For this review, take the finished solid that the model builds, in its own axes (mm). Face numbers are marked on the shaded views. A direction names the side the tool comes from. Round coordinates to 2 decimals unless told otherwise and drop trailing zeros. Write each loop counter-clockwise with the first axis right and the second up, starting at its lowest first coordinate (ties: lowest second). Pieces come first, ordered by that corner, then holes. Notation, with made-up numbers: (27, -14.75) -> (63, -14.75) arc R21 ccw to (63, 24.25) -> close; hole circle Ø9 at (4, -31). An arc over 180 degrees is marked (long way). Answer in a Markdown table with one row per item.
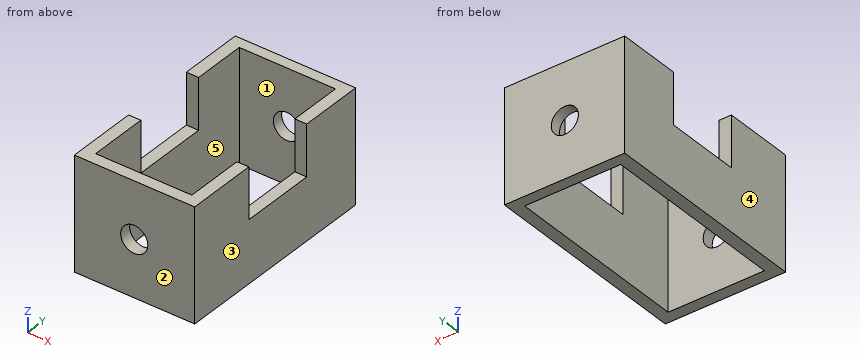
from build123d import *

# Parameters (mm, degrees)
F0_W     = 106.1013787985
F0_H     = 185.8578324318
F1_DEPTH = 99.4051918387
F2_R     = 11.9577926149
F3_DEPTH = 185.8588324318
F4_W     = 66.8169781566
F4_H     = 44.8713488877
F5_DEPTH = 106.1023787985
F6_W     = 84.8165526986
F6_H     = 165.8911928535
F7_DEPTH = 99.4061918387


with BuildPart() as f1:
    # F0 (on Top) → F1 (new body)
    with BuildSketch(Plane.XY):
        with Locations((-35.3671237826, 0)):
            Rectangle(F0_W, F0_H)
    extrude(amount=F1_DEPTH)

    # F2 (on face) → F3 (cut, through all)
    with BuildSketch(Plane.XZ.offset(92.9289162159)):
        with Locations((-35.6283932924, 49.7025959194)):
            Circle(F2_R)
    extrude(amount=-F3_DEPTH, mode=Mode.SUBTRACT)

    # F4 (on face) → F5 (cut, through all)
    with BuildSketch(Plane(origin=(-88.4178131819, 0, 0), x_dir=(0, -1, 0), z_dir=(-1, 0, 0))):
        with Locations((-3.043372184, 76.9695173949)):
            Rectangle(F4_W, F4_H)
    extrude(amount=-F5_DEPTH, mode=Mode.SUBTRACT)

    # F6 (on face) → F7 (cut, through all)
    with BuildSketch(Plane.XY.offset(99.4051918387)):
        with Locations((-35.2126248181, 0.4157535732)):
            Rectangle(F6_W, F6_H)
    extrude(amount=-F7_DEPTH, mode=Mode.SUBTRACT)


solid = f1.part
1) Mouldability with a two-part tool opening along X and no side actions: class the marked faces 1, 2 and 3 as pulls with the +X half, pulls with the -X half, needs draft (parallel to the pull), parting line crosses it, or undercut.
Solved:
| item | result |
|---|---|
| face 1 | undercut |
| face 2 | needs draft |
| face 3 | pulls with the +X half |
2) Clearance check with flat-ended pins moving along their axes: pin 1 Ø10 at (y, z) = (21, 64) entering from +X; pin 2 Ø8.5 at (x, y) = (14, 4) entering from +Z. State where each tip first meets the part, or that it passes through.
Solved:
| item | result |
|---|---|
| pin 1 | through |
| pin 2 | z = 54.53 |
3) For the marked faces 4 and 5, list the 3-axis set-ups (+Z, -Z, +X, -X, +Y, -Y) from which the entire face can be reached by the end or side of a thin tool; tool diameter is ignored.
Solved:
| item | result |
|---|---|
| face 4 | +Z, -Z, -X, +Y, -Y |
| face 5 | +Z, -Z |
4) Consider section C-C on y = 47.5. State the section outline as (x, z) points, then the cut area to 3 significant figures.
Solved:
| item | result |
|---|---|
| outline | (-88.42, 0) -> (-77.62, 0) -> (-77.62, 99.41) -> (-88.42, 99.41) -> close; (7.2, 0) -> (17.68, 0) -> (17.68, 99.41) -> (7.2, 99.41) -> close |
| area | 2,120 mm² |
5) For line 1 (X direction, y = -2.5, z = 33.5); line 2 (Y direction, x = -62.5, z = 6); line 3 (Z direction, x = 12, y = 1), list the stretches that pass through material, from the lowest coordinate up. Write a range as [from, to].
Solved:
| item | result |
|---|---|
| line 1 | [-88.42, -77.62], [7.2, 17.68] |
| line 2 | [-92.93, -82.53], [83.36, 92.93] |
| line 3 | [0, 54.53] |
6) Consider section A-A on x = -20.5. State the section outline as (y, z) points.
Solved:
| item | result |
|---|---|
| outline | (-92.93, 0) -> (-82.53, 0) -> (-82.53, 99.41) -> (-92.93, 99.41) -> close; (83.36, 0) -> (92.93, 0) -> (92.93, 99.41) -> (83.36, 99.41) -> close |
7) Consider section B-B on z = 79. State the section outline as (x, y) points, then the cut area to 3 significant figures.
Solved:
| item | result |
|---|---|
| outline | (-88.42, -92.93) -> (17.68, -92.93) -> (17.68, -30.37) -> (7.2, -30.37) -> (7.2, -82.53) -> (-77.62, -82.53) -> (-77.62, -30.37) -> (-88.42, -30.37) -> close; (-88.42, 36.45) -> (-77.62, 36.45) -> (-77.62, 83.36) -> (7.2, 83.36) -> (7.2, 36.45) -> (17.68, 36.45) -> (17.68, 92.93) -> (-88.42, 92.93) -> close |
| area | 4,230 mm² |
8) Consider section D-D on x = -39.5. State the section outline as (y, z) points, then the cut area to 3 significant figures.
Solved:
| item | result |
|---|---|
| outline | (-92.93, 0) -> (-82.53, 0) -> (-82.53, 38.39) -> (-92.93, 38.39) -> close; (-92.93, 61.02) -> (-82.53, 61.02) -> (-82.53, 99.41) -> (-92.93, 99.41) -> close; (83.36, 0) -> (92.93, 0) -> (92.93, 38.39) -> (83.36, 38.39) -> close; (83.36, 61.02) -> (92.93, 61.02) -> (92.93, 99.41) -> (83.36, 99.41) -> close |
| area | 1,530 mm² |
